The listing builds one solid part. Answer for the finished solid, in the listing's coordinates (mm). Face numbers are marked on the shaded views. A direction names the side the tool comes from. Give positions to 0.01 mm unless a question says otherwise; leave off trailing zeros. Order: outer loops, then holes, each group sorted by start corner. A loop starts at its lowest first (then second) coordinate and runs counter-clockwise, first axis right, second up.
```python
from build123d import *

# Parameters (mm, degrees)
F0_W     = 101.6
F0_H     = 101.6
F1_DEPTH = 101.6
F2_W     = 101.6
F2_H     = 76.2
F3_DEPTH = 63.5
F4_W     = 50.8
F4_H     = 19.05
F5_DEPTH = 76.2
F7_DEPTH = 25.4
F8_W     = 25.4
F8_H     = 25.4
F9_DEPTH = 25.4


with BuildPart() as f1:
    # F0 (on Front) → F1 (new body)
    with BuildSketch(Plane.XZ):
        with Locations((15.095475, -19.266974)):
            Rectangle(F0_W, F0_H)
    extrude(amount=F1_DEPTH)

    # F2 (on face) → F3 (cut)
    with BuildSketch(Plane.XZ.offset(101.6)):
        with Locations((15.095475, -6.566974)):
            Rectangle(F2_W, F2_H)
    extrude(amount=-F3_DEPTH, mode=Mode.SUBTRACT)

    # F4 (on face) → F5 (cut)
    with BuildSketch(Plane.XY.offset(31.533026)):
        with Locations((15.095475, -28.575)):
            Rectangle(F4_W, F4_H)
    extrude(amount=-F5_DEPTH, mode=Mode.SUBTRACT)

    # F6 (on face) → F7 (cut)
    with BuildSketch(Plane.XY.offset(-44.666974)):
        Polygon((-35.704525, -76.2), (-35.704525, -101.6), (-10.304525, -101.6), align=None)
        Polygon((65.895475, -76.2), (40.495475, -101.6), (65.895475, -101.6), align=None)
    extrude(amount=-F7_DEPTH, mode=Mode.SUBTRACT)

    # F8 (on face) → F9 (cut)
    with BuildSketch(Plane.XY.offset(-44.666974)):
        with Locations((15.095475, -63.5)):
            Rectangle(F8_W, F8_H)
    extrude(amount=-F9_DEPTH, mode=Mode.SUBTRACT)


solid = f1.part
```
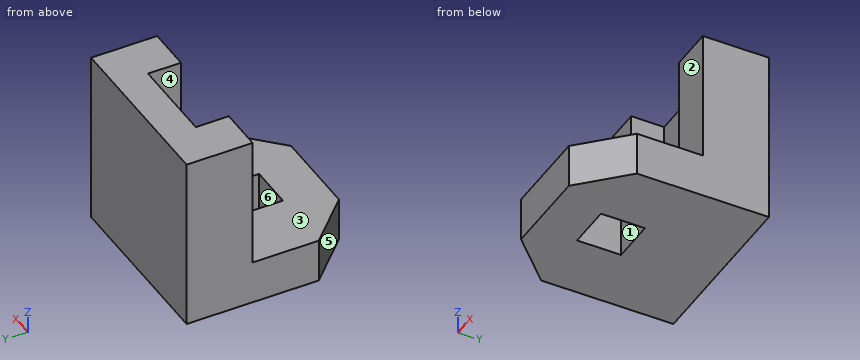
1) Find section C-C (x = 6). Write down the section's boundary in (y, z).
Geometry says:
outline: (-101.6, -70.07) - (-76.2, -70.07) - (-76.2, -44.67) - (-101.6, -44.67) - close; (-50.8, -70.07) - (0, -70.07) - (0, 31.53) - (-19.05, 31.53) - (-19.05, -44.67) - (-50.8, -44.67) - close
2) Find section B-B (y = -66.5). Write down the section's boundary in (x, z).
Geometry says:
outline: (-35.7, -70.07) - (2.4, -70.07) - (2.4, -44.67) - (-35.7, -44.67) - close; (27.8, -70.07) - (65.9, -70.07) - (65.9, -44.67) - (27.8, -44.67) - close
3) Find section D-D (z = -22). Write down the section's boundary in (x, y).
Geometry says:
outline: (-35.7, -38.1) - (-10.3, -38.1) - (-10.3, -19.05) - (40.5, -19.05) - (40.5, -38.1) - (65.9, -38.1) - (65.9, 0) - (-35.7, 0) - close
4) A tool of negligible diameter and unlimited length cuts with its end or side. For the marked faces 4, 5 and 6, from which of +Z, -Z, +X, -X, +Y, -Y can it reach the whole face along a straight path? Write none if from no direction.
Geometry says:
face 4: +Z, -Y
face 5: +Z, -Z, -X, -Y
face 6: +Z, -Z
5) Given P1, Ø3, axis at x = 31, y = -63, coming from the +Z side; P2, Ø20.5, axis at x = -22, z = -5.5, coming from the -Y side; P3, Ø4, axis at x = 29, z = -0.5, coming from the -Y side, each flat-ended and moving along its own axis, determine where each tip first touches the part or whether it passes through.
Geometry says:
P1: stops at z = -44.67
P2: stops at y = -38.1
P3: stops at y = -19.05
6) Straight lines are drawn through the part: probe 1 along Y at (x, z) = (24, -53); probe 2 along X at (y, z) = (-61, -60); probe 3 along X at (y, z) = (-32, 14). For each, find the intervals that lie inside material, in ascending order.
Geometry says:
probe 1: y = -101.6 to -76.2, -50.8 to 0
probe 2: x = -35.7 to 2.4, 27.8 to 65.9
probe 3: x = -35.7 to -10.3, 40.5 to 65.9
7) Find section A-A (z = -55.5). Write down the section's boundary in (x, y), then the cut area to 3 significant figures.
Geometry says:
outline: (-35.7, -76.2) - (-10.3, -101.6) - (40.5, -101.6) - (65.9, -76.2) - (65.9, 0) - (-35.7, 0) - close; hole (2.4, -76.2) - (27.8, -76.2) - (27.8, -50.8) - (2.4, -50.8) - close
area: 9,030 mm2
8) For a pull along Y with two mould halves and no side action, classify the marked faces 1, 2 and 3 as +Y half, -Y half, draft (parallel to the pull), parting line (faces both ways), or undercut.
Geometry says:
face 1: undercut
face 2: -Y half
face 3: draft
